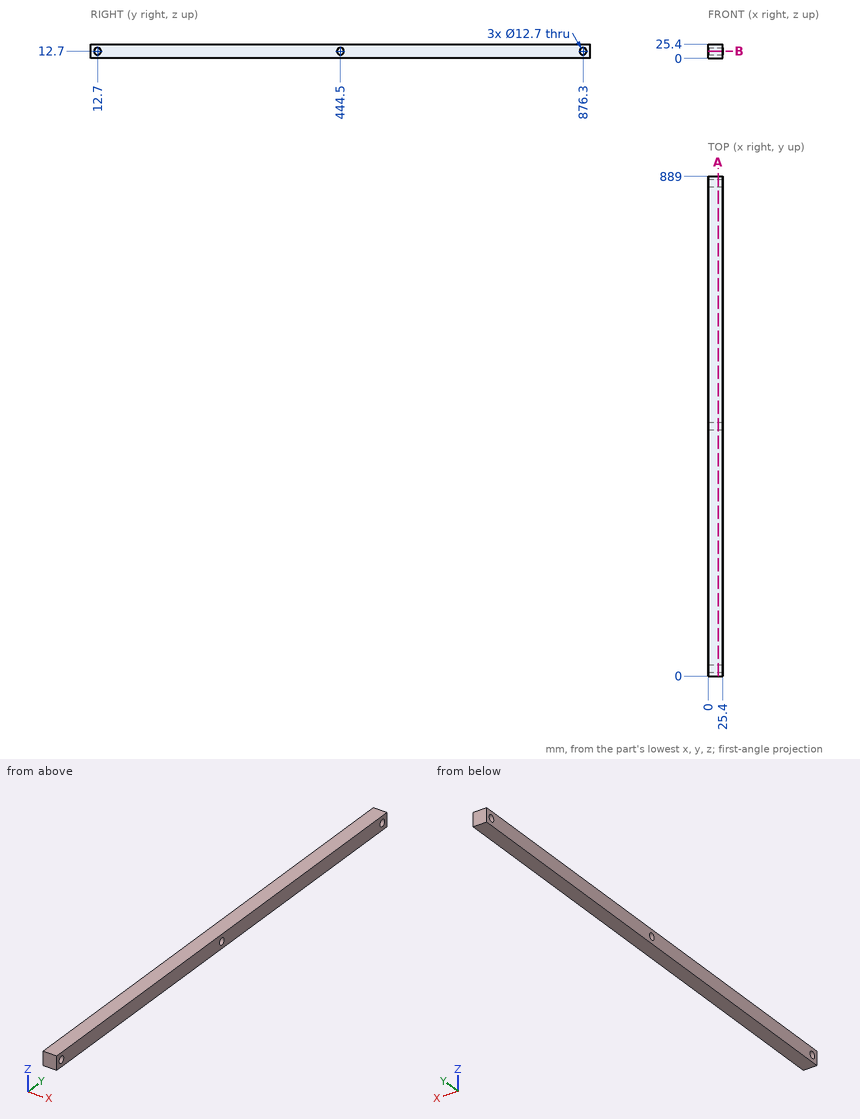
Study the drawing (mm; zero at the part's minimum x, y, z) and answer. Give positions to 0.01 mm unless a question says otherwise; leave off trailing zeros. Loops run counter-clockwise (first coordinate to the right, second up) from the corner with the lowest first, then second, coordinate; pieces in that order, holes last. Notation, with made-up numbers: (85, 58) - (136, 58) arc R30 ccw to (136, 91) - close; hole circle Ø10 at (-3.5, 52.25). An arc over 180 degrees is marked (long way). Use CSV: the item, a comma, the result in double quotes. Start each with the question number.
(1) This flat-tipped pin is pushed along its axis until it touches: pin 1 (8 mm diameter, centred on x = 22.5, z = 8.5, fed in from -Y). Where does it stop, or does it pass through?
(2) Find section A-A, the plane x = 17.5. Determine the outline of the cut face in (y, z).
(3) Find the intervals of material crossed by L1, parallel to Y at x = 7.25, z = 13.25; L2, parallel to Z at x = 5.5, y = 12.7; L3, parallel to Y at x = 23, z = 8, in increasing order.
(4) Find section B-B, the plane z = 12.7. Determine the outline of the cut face in (x, y), plus the area to 3 significant figures.
Results found:
1,pin 1,"y = 0"
2,outline,"(0, 0) - (889, 0) - (889, 25.4) - (0, 25.4) - close; hole circle Ø12.7 at (12.7, 12.7); hole circle Ø12.7 at (444.5, 12.7); hole circle Ø12.7 at (876.3, 12.7)"
3,L1,"0 to 6.37, 19.03 to 438.17, 450.83 to 869.97, 882.63 to 889"
3,L2,"0 to 6.35, 19.05 to 25.4"
3,L3,"0 to 8.43, 16.97 to 440.23, 448.77 to 872.03, 880.57 to 889"
4,outline,"(0, 0) - (25.4, 0) - (25.4, 6.35) - (0, 6.35) - close; (0, 19.05) - (25.4, 19.05) - (25.4, 438.15) - (0, 438.15) - close; (0, 450.85) - (25.4, 450.85) - (25.4, 869.95) - (0, 869.95) - close; (0, 882.65) - (25.4, 882.65) - (25.4, 889) - (0, 889) - close"
4,area,"21,600 mm^2"
